Autodesk Inventor part; units mm, degrees
ref_plane "YZ Plane" through (0, 0, 0) normal (1, 0, 0) x (0, 1, 0)
ref_plane "XZ Plane" through (0, 0, 0) normal (0, 1, 0) x (-1, 0, 0)
ref_plane "XY Plane" through (0, 0, 0) normal (0, 0, 1) x (1, 0, 0)
sketch "Эскиз1" plane through (0, 0, 0) normal (0, 0, 1) x (1, 0, 0)
  line L0 (0, 0) -> (0, 15)
  line L1 (0, 12.5) -> (3, 12.5)
  line L2 (1.7154, 2) -> (4.0415, 2)
  line L3 (2.5, 5) -> (4.0415, 5)
  line L4 (2.5, 6.5) -> (3, 6.5)
  line L5 (0, 0) -> (0.315, 0)
  line L6 (2.5, 6.5) -> (2.5, 5)
  line L7 (3, 12.5) -> (3, 6.5)
  line L8 (0.315, 0) -> (1.7154, 2)
  line L9 (4.0415, 5) -> (4.0415, 2)
  line L10 (0, 12.5) -> (0, 0)
  dimension "d0" = 15
  dimension "d1" = 12.5
  dimension "d2" = 10.5
  dimension "d3" = 7.5
  dimension "d4" = 6
  dimension "d6" = 5
  dimension "d7" = 6
  dimension "d8" = 125
  dimension "d11" = 8.083
  dimension "d44" = 0.63
revolve "Вращение1" add sketch "Эскиз1" angle 360 about axis through (0, 0, 0) along (0, 1, 0)
chamfer "Фаска1" distance 0.25 angle 45 2 edges at (-3, 12.5, 0) (-3, 6.5, 0)
thread "Резьба1"
sketch "Эскиз2" plane through (0, 12.5, 0) normal (0, 1, 0) x (1, 0, 0)
  point P0 (0, 0)
  point P1 (0, 0)
sketch "Эскиз3" plane through (0, 0, 0) normal (0, -1, 0) x (1, 0, 0)
  point P0 (0, 0)
  point P1 (0, 0)
hole "Отверстие1" at (0, 12.5, 0) direction (0, -1, 0) diameter 1 depth 12 tip angle 130
hole "Отверстие2" at (0, 12.5, 0) direction (0, -1, 0) diameter 2 depth 10.8 tip angle 130
chamfer "Фаска2" distance 0.2 angle 45 1 edges at (0, 12.5, -1)
hole "Отверстие3" at (0, 0, 0) direction (0, 1, 0) diameter 0.25 depth 0.5
sketch "Эскиз4" plane through (0, 2, 0) normal (0, -1, 0) x (1, 0, 0)
  circle A0 centre (0, 0) radius 0.125
  circle A1 centre (0, 0) radius 4.0415
  line L0 (4.0415, 0) -> (2.0208, -3.5)
  line L1 (2.0208, -3.5) -> (-2.0207, -3.5)
  line L2 (-2.0207, -3.5) -> (-4.0415, 0)
  line L3 (-4.0415, 0) -> (-2.0208, 3.5)
  line L4 (-2.0208, 3.5) -> (2.0207, 3.5)
  line L5 (2.0207, 3.5) -> (4.0415, 0)
extrude "Выдавливание1" cut sketch "Эскиз4" against normal blind 3 contours L5 A1 | A1 L0 | L4 A1 | A1 L1 | L3 A1 | A1 L2
properties part number "nozzle-0,25"
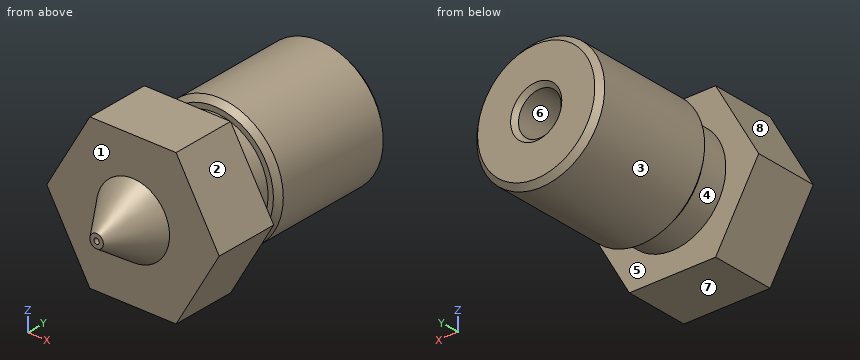
Read the model definition and answer for the solid it produces. Units are mm, in the model's axes. Face numbers are marked on the shaded views. A direction names the side the tool comes from. Coordinates: 2 decimals unless noted, no trailing zeros. Loops run counter-clockwise (first coordinate to the right, second up) from the corner with the lowest first, then second, coordinate; pieces in that order, holes last.
Q1. Which of the six approach directions +Z, -Z, +X, -X, +Y, -Y give full straight-line access (tool end or side, diameter ignored) to the marked faces 1, 2, 3 and 4?
Q2. Consider probe 1 along X at (y, z) = (11.25, 0); probe 2 along Z at (x, y) = (0, 4); probe 3 along Y at (x, z) = (-2.5, 0.75). Determine where each line is inside the solid, lowest interval first.
Q3. The part is cut by section C-C on y = 5.75. Write down the section's boundary in (x, z).
Q4. Each of these flat-tipped pins is pushed along its axis until it touches: pin 1 Ø2 at (x, z) = (1.5, 1.5) entering from -Y; pin 2 Ø2 at (y, z) = (7, -1.5) entering from -X; pin 3 Ø2 at (x, z) = (-0.5, 1) entering from +Y; pin 4 Ø1.5 at (x, y) = (0.5, 11) entering from -Z. Where does it stop, or does it pass through?
Q5. The part is cut by section A-A on y = 2.5. Write down the section's boundary in (x, z), and give its area (3 significant figures).
Q6. The mould has two halves that part along Z. Classify the marked faces 5, 6, 7 and 8: +Z half, -Z half, draft (parallel to the pull), parting line (faces both ways), or undercut.
Q7. The part is cut by section B-B on y = 9.5. Write down the section's boundary in (x, z).
Results below:
1. face 1: -Y
1. face 2: +Z, +X, +Y, -Y
1. face 3: +Y
1. face 4: none
2. probe 1: x = -3 to -1, 1 to 3
2. probe 2: z = -3.5 to -1, 1 to 3.5
2. probe 3: y = 2 to 5, 6.5 to 12.5
3. outline: circle Ø5 at (0, 0); hole circle Ø2 at (0, 0)
4. pin 1: stops at y = 1.15
4. pin 2: stops at x = -2.96
4. pin 3: stops at y = 12.5
4. pin 4: stops at z = -3
5. outline: (-4.04, 0) - (-2.02, -3.5) - (2.02, -3.5) - (4.04, 0) - (2.02, 3.5) - (-2.02, 3.5) - close; hole circle Ø2 at (0, 0)
5. area: 39.3 mm2
6. face 5: draft
6. face 6: undercut
6. face 7: -Z half
6. face 8: +Z half
7. outline: circle Ø6 at (0, 0); hole circle Ø2 at (0, 0)
